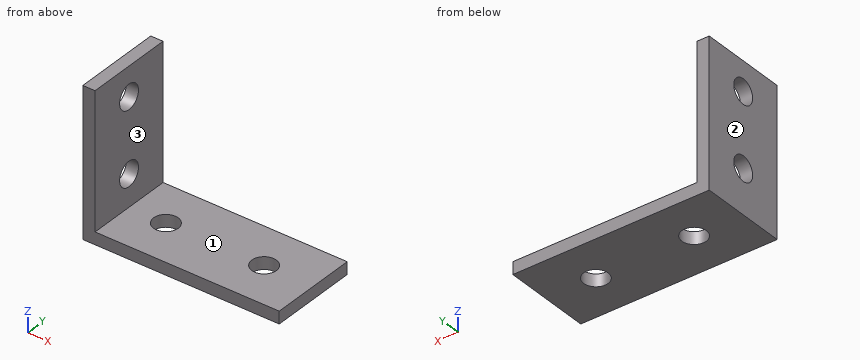
```python
from build123d import *

# Parameters (mm, degrees)
BOSS_EXTRUDE1_DEPTH         = 22.86
F_1_4_0_25_DIAMETER_HOLE1_D = 6.35
F_1_4_0_25_DIAMETER_HOLE2_D = 6.35


with BuildPart() as part:
    # Sketch1 → Boss-Extrude1 (new body)
    with BuildSketch(Plane(origin=(0, 0, 0), x_dir=(1, 0, 0), z_dir=(0, 1, 0))):
        Polygon((0, 0), (0, 38.1), (50.8, 38.1), (50.8, 34.925), (3.175, 34.925), (3.175, 0), align=None)
    extrude(amount=BOSS_EXTRUDE1_DEPTH)

    # 1/4 (0.25) Diameter Hole1 (through all)
    with Locations(Plane(origin=(3.175, 0, 0), x_dir=(0, 0, -1), z_dir=(1, 0, 0))):
        with Locations((7.62, 11.43), (26.67, 11.43)):
            Hole(F_1_4_0_25_DIAMETER_HOLE1_D / 2)

    # 1/4 (0.25) Diameter Hole2 (through all)
    with Locations(Plane(origin=(0, 0, -38.1), x_dir=(-1, 0, 0), z_dir=(0, 0, -1))):
        with Locations((-38.1, 11.43), (-12.7, 11.43)):
            Hole(F_1_4_0_25_DIAMETER_HOLE2_D / 2)


solid = part.part
```
Can you work these out from the model? Positions are in its coordinate system, mm. Face numbers are marked on the shaded views. Coordinates: 2 decimals unless noted, no trailing zeros. Loops run counter-clockwise (first coordinate to the right, second up) from the corner with the lowest first, then second, coordinate; pieces in that order, holes last.
Item 1: Suppose I cut it at B-B (y = 11.43). Please give me the cut outline in (x, z) (3 decimals).
Answers below:
outline: (0, -38.1) - (9.525, -38.1) - (9.525, -34.925) - (3.175, -34.925) - (3.175, -29.845) - (0, -29.845) - close; (0, -23.495) - (3.175, -23.495) - (3.175, -10.795) - (0, -10.795) - close; (0, -4.445) - (3.175, -4.445) - (3.175, 0) - (0, 0) - close; (15.875, -38.1) - (34.925, -38.1) - (34.925, -34.925) - (15.875, -34.925) - close; (41.275, -38.1) - (50.8, -38.1) - (50.8, -34.925) - (41.275, -34.925) - close
Item 2: Suppose I cut it at C-C (x = 14). Please give me the cut outline in (y, z) (3 decimals), then the cut area to 3 significant figures.
Answers below:
outline: (0, -38.1) - (8.533, -38.1) - (8.533, -34.925) - (0, -34.925) - close; (14.327, -38.1) - (22.86, -38.1) - (22.86, -34.925) - (14.327, -34.925) - close
area: 54.2 mm2
Item 3: If we mould it in two halves opening along X, with no side actions, what happens to the marked faces 1, 2 and 3? For each: released by +X, released by -X, zero draft, split by the parting line, or undercut.
Answers below:
face 1: zero draft
face 2: released by -X
face 3: released by +X
Item 4: Please list where these lines run through material, in increasing order: L1, parallel to Y at x = 12.7, z = -37 (3 decimals); L2, parallel to Z at x = 12, y = 15.75 (3 decimals); L3, parallel to X at y = 5, z = -33.5 (3 decimals).
Answers below:
L1: y = 0 to 8.255, 14.605 to 22.86
L2: z = -38.1 to -34.925
L3: x = 0 to 3.175
Item 5: Suppose I cut it at D-D (y = 9). Please give me the cut outline in (x, z) (3 decimals).
Answers below:
outline: (0, -38.1) - (10.657, -38.1) - (10.657, -34.925) - (3.175, -34.925) - (3.175, -28.713) - (0, -28.713) - close; (0, -24.627) - (3.175, -24.627) - (3.175, -9.663) - (0, -9.663) - close; (0, -5.577) - (3.175, -5.577) - (3.175, 0) - (0, 0) - close; (14.743, -38.1) - (36.057, -38.1) - (36.057, -34.925) - (14.743, -34.925) - close; (40.143, -38.1) - (50.8, -38.1) - (50.8, -34.925) - (40.143, -34.925) - close
Item 6: I'm going to push flat-ended pins straight in: pin 1 (8 mm diameter, centred on x = 28.5, y = 3.5, fed in from +Z) (3 decimals); pin 2 (1.5 mm diameter, centred on y = 10.5, z = -21.5, fed in from +X) (3 decimals). Where does each tip first touch, or does it pass through?
Answers below:
pin 1: stops at z = -34.925
pin 2: stops at x = 3.175
Item 7: Suppose I cut it at A-A (z = -7.62). Please give me the cut outline in (x, y) (3 decimals).
Answers below:
outline: (0, 0) - (3.175, 0) - (3.175, 8.255) - (0, 8.255) - close; (0, 14.605) - (3.175, 14.605) - (3.175, 22.86) - (0, 22.86) - close
